Model file for the job. Use its own axes, mm. A direction names the side the tool comes from. Round coordinates to 2 decimals unless told otherwise and drop trailing zeros. Order: outer loops, then holes, each group sorted by start corner. A loop starts at its lowest first (then second) coordinate and runs counter-clockwise, first axis right, second up. Notation, with made-up numbers: (-15.75, 57.5) - (-7.75, 57.5) arc R15 cw to (-7.75, 67.5) - close; hole circle Ø11 at (35.5, 86.5). An arc over 180 degrees is marked (long way). Answer as CSV lines item,"result". Start each with the question number.
1. Band-saw the part on A-A on x = 0. List the corners of the cut face in (y, z), then the cut area to 3 significant figures.
2. Pin check, flat tips, straight feed: pin 1 Ø5 at (x, z) = (-4.5, -11) entering from -Y; pin 2 Ø1 at (y, z) = (4, -25.5) entering from -X; pin 3 Ø6 at (x, y) = (2.5, 2) entering from +Z; pin 4 Ø1 at (x, z) = (2, -11.5) entering from -Y. Stop position of each tip, or through.
3. Band-saw the part on C-C on z = -19. List the corners of the cut face in (x, y).
4. Wall check: line 1 along Z through (x, y) = (5, -0.5); line 2 along X through (y, z) = (1.25, -12); line 3 along X through (y, z) = (-0.25, -11.5). Give the ranges that are in metal, low to high. Write a range as [from, to].
5. Pull direction Z, two halves, no side cores. Call faces 1 (the face through (0, 0, -31)), 2 (the face through (3.796, -0.167, -28.493)), 3 (the face through (0.867, 3.905, -15.325)): released by +Z, released by -Z, zero draft, split by the parting line, or undercut.
6. 3-axis set-ups, long thin cutter, end or side, ignore diameter. For faces 4 (the face through (0, 0, 0)), 5 (the face through (-1.42, -3.92, -3)): which of +Z, -Z, +X, -X, +Y, -Y reach the whole face in a straight line?
Autodesk Inventor part; units mm, degrees
ref_plane "YZ Plane" through (0, 0, 0) normal (1, 0, 0) x (0, 1, 0)
ref_plane "XZ Plane" through (0, 0, 0) normal (0, 1, 0) x (-1, 0, 0)
ref_plane "XY Plane" through (0, 0, 0) normal (0, 0, 1) x (1, 0, 0)
sketch "Sketch1" plane through (0, 0, 0) normal (0, 0, 1) x (1, 0, 0)
  circle A0 centre (0, 0) radius 6
  dimension "d0" = 12
extrude "Extrusion1" add sketch "Sketch1" against normal blind 3
chamfer "Chamfer1" distance 0.5 angle 45 1 edges at (-6, 0, 0) measured on face at (5.9805, -0.4828, -2)
sketch "Sketch2" plane through (0, 0, -3) normal (0, 0, -1) x (-1, 0, 0)
  circle A0 centre (0, 0) radius 4
  dimension "d6" = 8
extrude "Extrusion2" add sketch "Sketch2" along normal blind 25
sketch "Sketch3" plane through (0, 0, -28) normal (0, 0, -1) x (-1, 0, 0)
  circle A0 centre (0, 0) radius 3.8
  dimension "d9" = 7.6
extrude "Extrusion3" add sketch "Sketch3" along normal blind 1
sketch "Sketch4" plane through (0, 0, -29) normal (0, 0, -1) x (-1, 0, 0)
  circle A0 centre (0, 0) radius 4
extrude "Extrusion4" add sketch "Sketch4" along normal blind 2
chamfer "Chamfer2" distance 0.5 angle 45 1 edges at (4, 0, -31)
properties part number "Bolt"
Reply:
1,outline,"(-6, -3) - (-4, -3) - (-4, -28) - (-3.8, -28) - (-3.8, -29) - (-4, -29) - (-4, -30.5) - (-3.5, -31) - (3.5, -31) - (4, -30.5) - (4, -29) - (3.8, -29) - (3.8, -28) - (4, -28) - (4, -3) - (6, -3) - (6, -0.5) - (5.5, 0) - (-5.5, 0) - (-6, -0.5) - close"
1,area,"259 mm2"
2,pin 1,"stops at y = -3.46"
2,pin 2,"stops at x = -1.94"
2,pin 3,"stops at z = 0"
2,pin 4,"stops at y = -3.71"
3,outline,"circle Ø8 at (0, 0)"
4,line 1,"z = [-3, 0]"
4,line 2,"x = [-3.8, 3.8]"
4,line 3,"x = [-3.99, 3.99]"
5,face 1,"released by -Z"
5,face 2,"undercut"
5,face 3,"zero draft"
6,face 4,"+Z, +X, -X, +Y, -Y"
6,face 5,"-Z"
